Geometry: see drawing. Coordinates: mm, zero at the bounding-box minimum. A direction names the side the tool comes from. Round coordinates to 2 decimals unless told otherwise and drop trailing zeros. Write each loop counter-clockwise with the first axis right and the second up, starting at its lowest first coordinate (ties: lowest second). Pieces come first, ordered by that corner, then holes. Notation, with made-up numbers: M 58.25,-5 L 86.25,-5 A8 cw 86.25,6 Z; hole C 65,-16 d7. An arc over 180 degrees is marked long. Use one line per item in the form item = value. Start each with the question number.
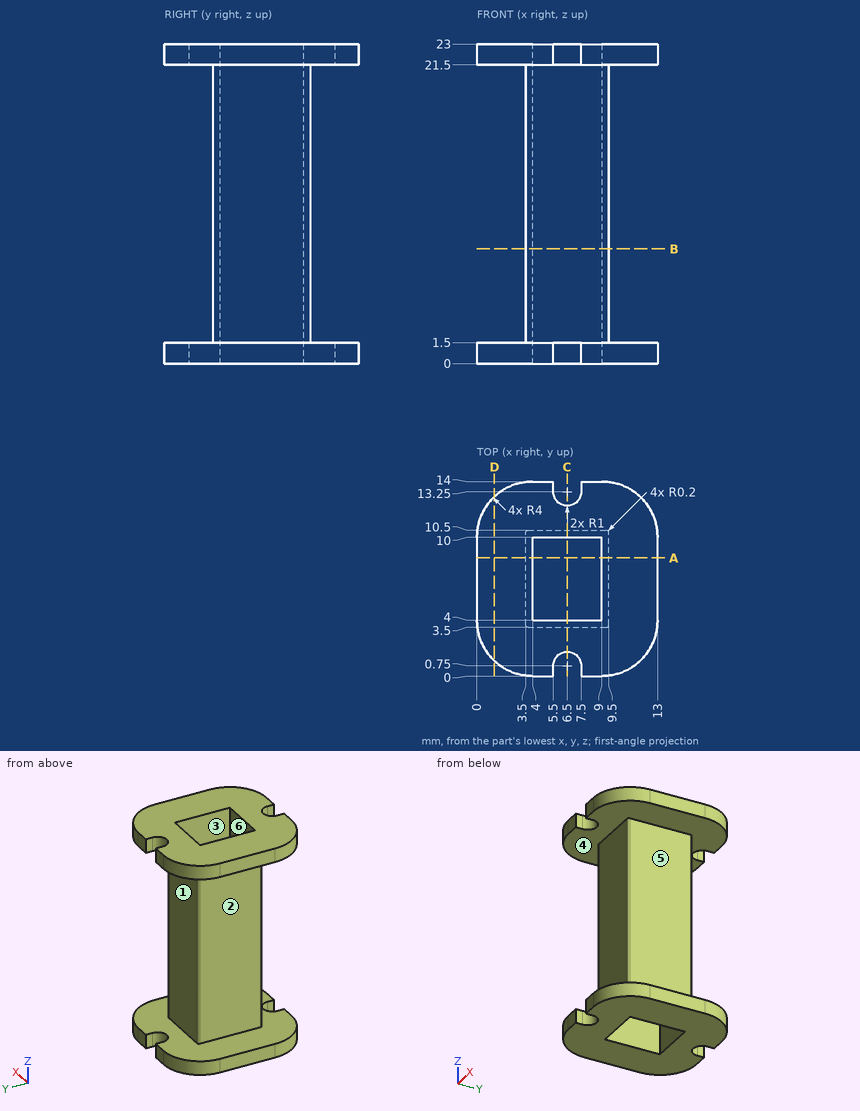
Item 1: Cut plane A-A (y = 8.5). Output: boundary loops of the cut face in (x, z), plus the area to 3 significant figures.
Item 2: Ray query, line 1 (Y direction, x = 6.5, z = 14.5); line 2 (Z direction, x = 11, y = 12.25); line 3 (X direction, y = 8, z = 19). Return the intervals inside material, ascending. Write a range as from..to.
Item 3: First-contact query: pin 1 (4 mm diameter, centred on x = 6.5, z = 10, fed in from -Y); pin 2 (5 mm diameter, centred on y = 11, z = 17.5, fed in from -X); pin 3 (1.5 mm diameter, centred on x = 6.5, z = 13.5, fed in from +Y). Flat tips, straight axial feed; report the tip coordinate or a pass-through.
Item 4: Cut plane C-C (x = 6.5). Output: boundary loops of the cut face in (y, z), plus the area to 3 significant figures.
Item 5: Cut plane B-B (z = 8.25). Output: boundary loops of the cut face in (x, y).
Item 6: Reachability of the marked faces 4, 5 and 6 from +Z, -Z, +X, -X, +Y, -Y: full face, straight path, thin tool, end or side. Return the list, or none.
Item 7: Draft query along Y for the marked faces 1, 2 and 3. Return one class per face: +Y half, -Y half, draft (parallel to the pull), parting line (faces both ways), or undercut.
Item 8: Cut plane D-D (x = 1.25). Output: boundary loops of the cut face in (y, z).
Final values:
q1.outline = M 0,0 L 4,0 L 4,23 L 0,23 L 0,21.5 L 3.5,21.5 L 3.5,1.5 L 0,1.5 Z; M 9,0 L 13,0 L 13,1.5 L 9.5,1.5 L 9.5,21.5 L 13,21.5 L 13,23 L 9,23 Z
q1.area = 44.0 mm^2
q2.line_1 = 3.5..4, 10..10.5
q2.line_2 = 0..1.5, 21.5..23
q2.line_3 = 3.5..4, 9..9.5
q3.pin_1 = 3.5
q3.pin_2 = 3.5
q3.pin_3 = 10.5
q4.outline = M 1.75,0 L 4,0 L 4,23 L 1.75,23 L 1.75,21.5 L 3.5,21.5 L 3.5,1.5 L 1.75,1.5 Z; M 10,0 L 12.25,0 L 12.25,1.5 L 10.5,1.5 L 10.5,21.5 L 12.25,21.5 L 12.25,23 L 10,23 Z
q4.area = 33.5 mm^2
q5.outline = M 3.5,3.7 A0.2 ccw 3.7,3.5 L 9.3,3.5 A0.2 ccw 9.5,3.7 L 9.5,10.3 A0.2 ccw 9.3,10.5 L 3.7,10.5 A0.2 ccw 3.5,10.3 Z; hole M 4,4 L 9,4 L 9,10 L 4,10 Z
q6.face_4 = none
q6.face_5 = +X, +Y, -Y
q6.face_6 = +Z, -Z
q7.face_1 = +Y half
q7.face_2 = draft
q7.face_3 = undercut
q8.outline = M 1.1,0 L 12.9,0 L 12.9,1.5 L 1.1,1.5 Z; M 1.1,21.5 L 12.9,21.5 L 12.9,23 L 1.1,23 Z
